Read the model definition and answer for the solid it produces. Units are mm, in the model's axes. Give positions to 0.01 mm unless a question says otherwise; leave off trailing zeros. Loops run counter-clockwise (first coordinate to the right, second up) from the corner with the lowest first, then second, coordinate; pieces in that order, holes last. Notation, with made-up numbers: (-11.5, -1.75) - (37.5, -1.75) arc R32 ccw to (37.5, 28.25) - close; hole circle Ø10 at (18.25, 1.5). An arc over 180 degrees is marked (long way). Use a Markdown table: item, result. Add a question column.
Item 1: A cutting plane is placed at D-D (z = 849.5). Determine the outline of the cut face in (x, y) (1 decimal).
Item 2: A cutting plane is placed at B-B (y = 0). Determine the outline of the cut face in (x, z).
Item 3: Each of these flat-tipped pins is pushed along its axis until it touches: P1, Ø5, axis at y = -5, z = 847.5, coming from the -X side; P2, Ø6, axis at x = 2, z = 798.5, coming from the -Y side; P3, Ø8, axis at x = 17.5, y = -11.5, coming from the +Z side; P4, Ø1.5, axis at x = 7, z = 641, coming from the -Y side. Where does it stop, or does it pass through?
Item 4: A cutting plane is placed at C-C (z = 228.6). Determine the outline of the cut face in (x, y) (1 decimal), plus the area to 3 significant figures.
Item 5: A cutting plane is placed at A-A (x = 0). Determine the outline of the cut face in (y, z), plus the area to 3 significant figures.
Item 6: Consider probe 1 along Z at (x, y) = (25.75, 0); probe 2 along Y at (x, z) = (-3, 640); probe 3 along X at (y, z) = (-1, 454). Determine where each line is inside the solid, lowest interval first. Write a range as [from, to].
from build123d import *

# Parameters (mm, degrees)
F0_R          = 30.1625
F0_R_2        = 25.4
F1_DEPTH      = 1016
F2_R          = 12.7
F3_DEPTH      = 31.1625001
F3_DEPTH_BACK = 31.1625001


with BuildPart() as f1:
    # F0 (on Top) → F1 (new body)
    with BuildSketch(Plane.XY):
        Circle(F0_R)
        Circle(F0_R_2, mode=Mode.SUBTRACT)
    extrude(amount=F1_DEPTH)

    # F2 (on Right) → F3 (cut, two sides)
    with BuildSketch(Plane.YZ) as f3_sk:
        with Locations((0, 228.6)):
            Circle(F2_R)
        with Locations((0, 787.4)):
            Circle(F2_R)
    extrude(amount=F3_DEPTH, mode=Mode.SUBTRACT)
    extrude(f3_sk.sketch, amount=-F3_DEPTH_BACK, mode=Mode.SUBTRACT)


solid = f1.part
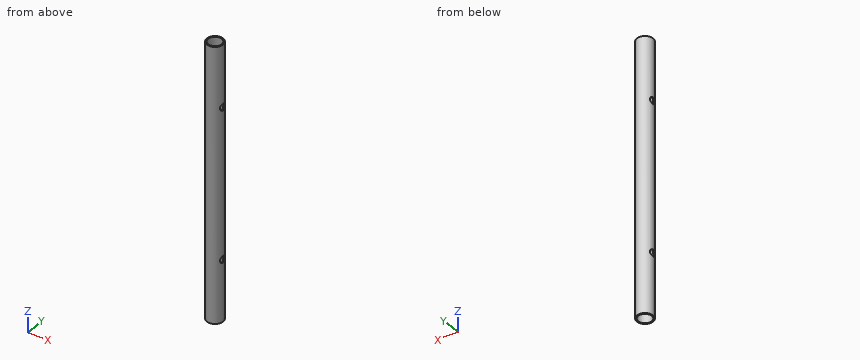
Geometry says:
| question | item | result |
|---|---|---|
| 1 | outline | circle Ø60.3 at (0, 0); hole circle Ø50.8 at (0, 0) |
| 2 | outline | (-30.16, 0) - (-25.4, 0) - (-25.4, 215.9) - (-30.16, 215.9) - close; (-30.16, 241.3) - (-25.4, 241.3) - (-25.4, 774.7) - (-30.16, 774.7) - close; (-30.16, 800.1) - (-25.4, 800.1) - (-25.4, 1016) - (-30.16, 1016) - close; (25.4, 0) - (30.16, 0) - (30.16, 215.9) - (25.4, 215.9) - close; (25.4, 241.3) - (30.16, 241.3) - (30.16, 774.7) - (25.4, 774.7) - close; (25.4, 800.1) - (30.16, 800.1) - (30.16, 1016) - (25.4, 1016) - close |
| 3 | P1 | x = -30.06 |
| 3 | P2 | y = -30.16 |
| 3 | P3 | through |
| 3 | P4 | y = -29.51 |
| 4 | outline | (-27.4, -12.7) arc R30.2 ccw to (27.4, -12.7) - (22, -12.7) arc R25.4 cw to (-22, -12.7) - close; (-27.4, 12.7) - (-22, 12.7) arc R25.4 cw to (22, 12.7) - (27.4, 12.7) arc R30.2 ccw to start |
| 4 | area | 580 mm² |
| 5 | outline | (-30.16, 0) - (-25.4, 0) - (-25.4, 1016) - (-30.16, 1016) - close; (25.4, 0) - (30.16, 0) - (30.16, 1016) - (25.4, 1016) - close |
| 5 | area | 9,680 mm² |
| 6 | probe 1 | [0, 215.9], [241.3, 774.7], [800.1, 1016] |
| 6 | probe 2 | [-30.01, -25.22], [25.22, 30.01] |
| 6 | probe 3 | [-30.15, -25.38], [25.38, 30.15] |
